For this review, use the dimensioned drawing (mm, ordinates from the lowest corner) and the shaded views. A direction names the side the tool comes from. Coordinates: 2 decimals unless noted, no trailing zeros. Order: outer loops, then holes, each group sorted by start corner. A loop starts at its lowest first (then second) coordinate and runs counter-clockwise, first axis right, second up. Notation, with made-up numbers: (85, 59) -> (104, 59) arc R6 cw to (104, 70) -> close; hole circle Ø9 at (-31, -36.5). An arc over 180 degrees is marked (long way). Use one line per item in the form item = value. Start each with the question number.
(1) Take a section at A-A (x = 6). State the section outline as (y, z) points (1 decimal).
(2) Insertion check: pin 1 Ø5 at (x, y) = (9, 2.5) entering from +Z; pin 2 Ø1 at (x, z) = (7.5, 2) entering from +Y; pin 3 Ø1 at (y, z) = (4.5, 5) entering from +X. Each pin has a flat end and moves straight along its axis. Give the tip position at first contact, or say it passes through.
(3) Take a section at B-B (y = 7). State the section outline as (x, z) points.
(4) Mouldability with a two-part tool opening along X and no side actions: class the marked faces 1, 2 and 3 as +X half, -X half, draft (parallel to the pull), parting line (faces both ways), or undercut.
(5) Take a section at D-D (y = 1.5). State the section outline as (x, z) points (1 decimal).
(6) Wall thickness on line 1 along X through (y, z) = (5.75, 1.5) (1 decimal); line 2 along X through (y, z) = (1.25, 0.5) (1 decimal); line 3 along X through (y, z) = (7.5, 5.5): over which ranges is each line inside the solid? List them lowest first.
(7) For the marked faces 4, 5 and 6, list the 3-axis set-ups (+Z, -Z, +X, -X, +Y, -Y) from which the entire face can be reached by the end or side of a thin tool; tool diameter is ignored.
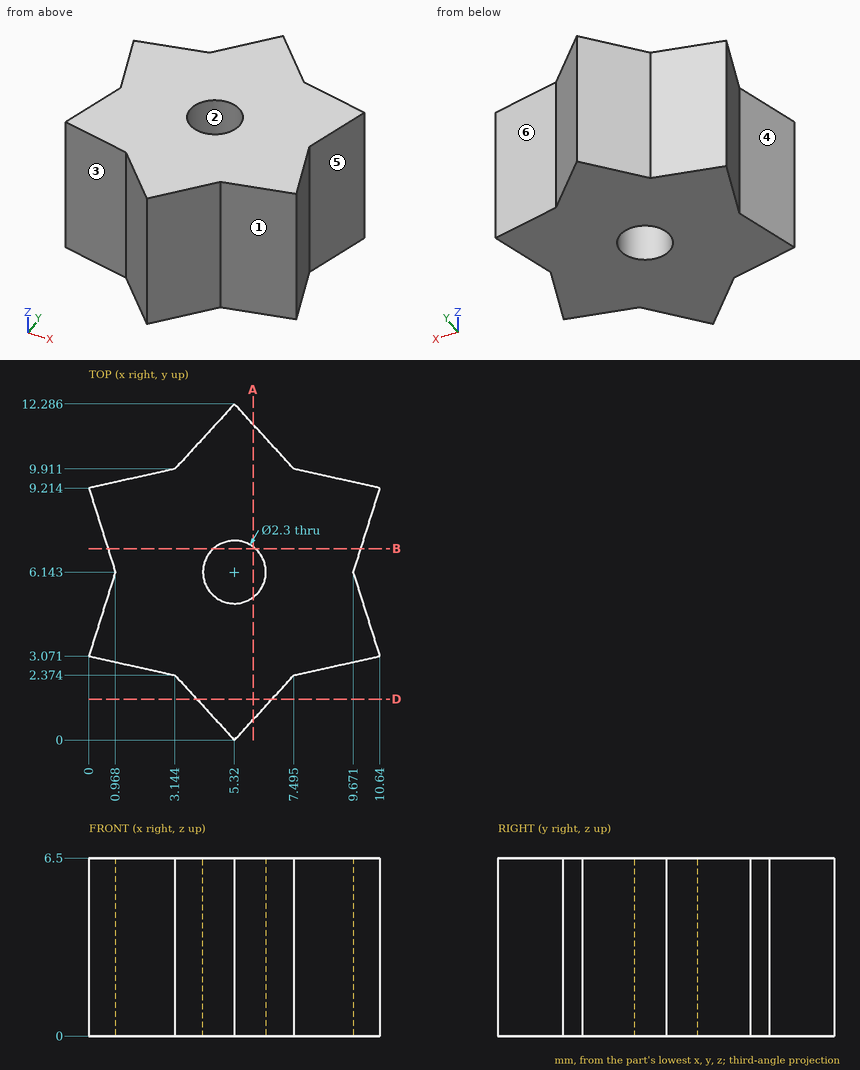
Findings:
q1.outline = (0.7, 0) -> (5.2, 0) -> (5.2, 6.5) -> (0.7, 6.5) -> close; (7.1, 0) -> (11.5, 0) -> (11.5, 6.5) -> (7.1, 6.5) -> close
q2.pin_1 = 6.5
q2.pin_2 = 10.45
q2.pin_3 = 10.35
q3.outline = (0.7, 0) -> (4.55, 0) -> (4.55, 6.5) -> (0.7, 6.5) -> close; (6.09, 0) -> (9.94, 0) -> (9.94, 6.5) -> (6.09, 6.5) -> close
q4.face_1 = +X half
q4.face_2 = undercut
q4.face_3 = -X half
q5.outline = (3.9, 0) -> (6.7, 0) -> (6.7, 6.5) -> (3.9, 6.5) -> close
q6.line_1 = 0.8 to 4.2, 6.4 to 9.8
q6.line_2 = 4.2 to 6.5
q6.line_3 = 0.54 to 10.1
q7.face_4 = +Z, -Z, -X
q7.face_5 = +Z, -Z, +X
q7.face_6 = +Z, -Z, +X, +Y
